```python
from build123d import *

# Parameters (mm, degrees)
F0_W     = 66.675
F0_H     = 63.5
F1_DEPTH = 50.8
F3_DEPTH = 66.675


with BuildPart() as f1:
    # F0 (on Front) → F1 (new body)
    with BuildSketch(Plane.XZ):
        with Locations((33.3375, 31.75)):
            Rectangle(F0_W, F0_H)
    extrude(amount=F1_DEPTH)

    # F2 (on face) → F3 (join)
    with BuildSketch(Plane.YZ.offset(66.675)):
        Polygon((-50.8, 15.875), (-50.8, 0), (0, 0), (0, 47.625), align=None)
    extrude(amount=F3_DEPTH)


solid = f1.part
```
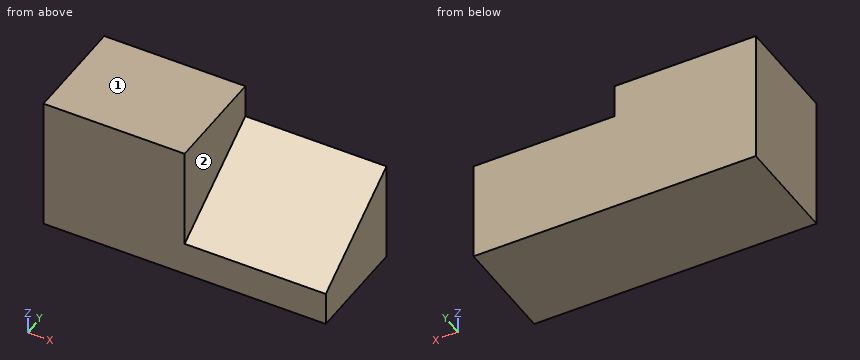
Model file for the job. Use its own axes, mm. Face numbers are marked on the shaded views. A direction names the side the tool comes from. Round coordinates to 2 decimals unless told otherwise and drop trailing zeros. Order: outer loops, then holes, each group sorted by start corner. A loop starts at its lowest first (then second) coordinate and runs counter-clockwise, first axis right, second up. Notation, with made-up numbers: M 73.25,44.25 L 112.25,44.25 A26 cw 112.25,70.25 Z; hole C -12.75,-20.5 d5. An arc over 180 degrees is marked long. Use CSV: the item, a comma, the result in double quotes.
Item 1: Pin check, flat tips, straight feed: pin 1 (1 mm diameter, centred on y = -28.5, z = 53.5, fed in from -X); pin 2 (5 mm diameter, centred on x = 70.5, y = -13.5, fed in from +Z); pin 3 (8 mm diameter, centred on x = 89.5, y = -31, fed in from +Z); pin 4 (10 mm diameter, centred on x = 98, y = -20, fed in from +Z). Stop position of each tip, or through.
Worked answers:
pin 1,"x = 0"
pin 2,"z = 40.75"
pin 3,"z = 30.75"
pin 4,"z = 38.25"
Item 2: Saw through at B-B (z = 31). List the corners of the cut face in (x, y) (3 decimals).
Worked answers:
outline,"M 0,-50.8 L 66.675,-50.8 L 66.675,-26.6 L 133.35,-26.6 L 133.35,0 L 0,0 Z"
Item 3: Which spindle directions (+Z, -Z, +X, -X, +Y, -Y) get a long thin tool onto all of the face, cutting with end or side? Do the marked faces 1 and 2. Say none if no direction does.
Worked answers:
face 1,"+Z, +X, -X, +Y, -Y"
face 2,"+Z, +X, -Y"
Item 4: Saw through at A-A (y = -21). List the corners of the cut face in (x, z) (3 decimals).
Worked answers:
outline,"M 0,0 L 133.35,0 L 133.35,34.5 L 66.675,34.5 L 66.675,63.5 L 0,63.5 Z"
Item 5: Probe probe 1 along X at (y, z) = (-39, 29.5) (3 decimals); probe 2 along Z at (x, y) = (110, -18.5); probe 3 along Y at (x, z) = (105, 32). List the from-to ranges inside material, lowest first.
Worked answers:
probe 1,"0 to 66.675"
probe 2,"0 to 36.06"
probe 3,"-25 to 0"
Item 6: Saw through at C-C (x = 79). List the corners of the cut face in (y, z) (3 decimals), plus the area to 3 significant figures.
Worked answers:
outline,"M -50.8,0 L 0,0 L 0,47.625 L -50.8,15.875 Z"
area,"1,610 mm²"
